```python
from build123d import *

# Parameters (mm, degrees)
F0_W     = 600
F0_H     = 300
F1_DEPTH = 10
F2_W     = 590.0000214577
F2_H     = 290.0000214577
F3_DEPTH = 5
F4_W     = 200
F4_H     = 150
F5_DEPTH = 30
F6_R     = 5
F7_R     = 20
F8_DEPTH = 10


with BuildPart() as f1:
    # F0 (on Front) → F1 (new body)
    with BuildSketch(Plane.XZ):
        with Locations((-100, 103.4820094705)):
            Rectangle(F0_W, F0_H)
    extrude(amount=F1_DEPTH)

    # F2 (on face) → F3 (cut)
    with BuildSketch(Plane.XZ.offset(10)):
        with Locations((-100, 103.4820094705)):
            Rectangle(F2_W, F2_H)
    extrude(amount=-F3_DEPTH, mode=Mode.SUBTRACT)

    # F4 (on face) → F5 (join)
    with BuildSketch(Plane.XZ.offset(5)):
        with Locations((-200, 125)):
            Rectangle(F4_W, F4_H)
    extrude(amount=-F5_DEPTH)

    # F6
    f6_edges = [f1.edges().sort_by_distance(p)[0] for p in [
        (-100, 0, 125),
        (-100, 12.5, 200),
        (-100, 25, 125),
        (-100, 12.5, 50),
        (-300, 0, 125),
        (-300, 12.5, 50),
        (-300, 25, 125),
        (-300, 12.5, 200),
        (-200, 0, 200),
        (-200, 0, 50),
    ]]
    fillet(f6_edges, radius=F6_R)

    # F7 (on face) → F8 (cut)
    with BuildSketch(Plane(origin=(0, 25, 0), x_dir=(-1, 0, 0), z_dir=(0, 1, 0))):
        with Locations((199.6024996042, 138.1175220013)):
            Circle(F7_R)
    extrude(amount=-F8_DEPTH, mode=Mode.SUBTRACT)


solid = f1.part
```
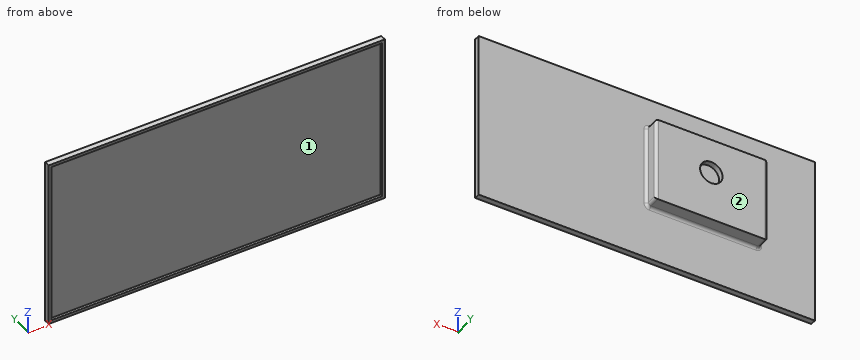
Could you check a few things on this model? Use its own coordinates, in mm. Face numbers are marked on the shaded views. Round coordinates to 2 decimals unless told otherwise and drop trailing zeros. Loops run counter-clockwise (first coordinate to the right, second up) from the corner with the lowest first, then second, coordinate; pieces in that order, holes last. Notation, with made-up numbers: (84, 55.5) -> (141, 55.5) arc R12 ccw to (141, 72.5) -> close; hole circle Ø9 at (-2.5, -26.75). An arc over 180 degrees is marked (long way). Put each result on its own line as item: value.
Q1. For pin 1 Ø12 at (x, z) = (-270.5, 138.5) entering from -Y; pin 2 Ø16.5 at (y, z) = (14.5, 150.5) entering from +X; pin 3 Ø12 at (x, z) = (-206.5, 132) entering from +Y, each with a flat end and sliding along its axis, tell me the tip position at first contact or that it passes through.
Checks:
pin 1: y = -5
pin 2: x = -100
pin 3: y = 15
Q2. Please list where these lines run through material, in increasing order: line 1 (Y direction, x = -263, z = 159.5); line 2 (Y direction, x = -9.5, z = 17); line 3 (Z direction, x = -279, y = 7.5). Write a range as from..to.
Checks:
line 1: -5..25
line 2: -5..0
line 3: 50..200
Q3. Thinking about a two-plate mould opening in Z: for the marked faces 1 and 2, which applies, pulls with the +Z half, pulls with the -Z half, needs draft (parallel to the pull), parting line crosses it, or undercut?
Checks:
face 1: undercut
face 2: needs draft
Q4. I want a section at D-D on z = 146. Write out the boundary of the cut face in (x, y), and give its area (3 significant figures).
Checks:
outline: (-400, -10) -> (-395, -10) -> (-395, -5) -> (195, -5) -> (195, -10) -> (200, -10) -> (200, 0) -> (-95, 0) arc R5 cw to (-100, 5) -> (-100, 20) arc R5 ccw to (-105, 25) -> (-181.22, 25) -> (-181.22, 15) -> (-217.98, 15) -> (-217.98, 25) -> (-295, 25) arc R5 ccw to (-300, 20) -> (-300, 5) arc R5 cw to (-305, 0) -> (-400, 0) -> close
area: 7,680 mm2
Q5. I want a section at A-A on z = 233. Write out the boundary of the cut face in (x, y), and give its area (3 significant figures).
Checks:
outline: (-400, -10) -> (-395, -10) -> (-395, -5) -> (195, -5) -> (195, -10) -> (200, -10) -> (200, 0) -> (-400, 0) -> close
area: 3,050 mm2
Q6. I want a section at B-B on x = 1.5. Write out the boundary of the cut face in (y, z).
Checks:
outline: (-10, -46.52) -> (0, -46.52) -> (0, 253.48) -> (-10, 253.48) -> (-10, 248.48) -> (-5, 248.48) -> (-5, -41.52) -> (-10, -41.52) -> close
Q7. I want a section at C-C on x = -232.5. Write out the boundary of the cut face in (y, z).
Checks:
outline: (-10, -46.52) -> (0, -46.52) -> (0, 45) arc R5 cw to (5, 50) -> (25, 50) -> (25, 200) -> (5, 200) arc R5 cw to (0, 205) -> (0, 253.48) -> (-10, 253.48) -> (-10, 248.48) -> (-5, 248.48) -> (-5, -41.52) -> (-10, -41.52) -> close
